from build123d import *

# Parameters (mm, degrees)
SKETCH007_R             = 3.5
SKETCH007_W             = 40
SKETCH007_H             = 65
PAD003_DEPTH            = 2
SKETCH017_W             = 44
SKETCH017_H             = 76
SKETCH017_W_2           = 40
SKETCH017_H_2           = 65
PAD009_DEPTH            = 12
SKETCH018_R             = 1
POCKET003_DEPTH         = 44
CHAMFER003_SIZE         = 5
CHAMFER004_SIZE         = 4
FILLET012_R             = 5
FILLET013_R             = 7
FILLET014_R             = 2
BODY001_ROLL_ANGLE      = 90
BODY001_PLACEMENT_ANGLE = 180


with BuildPart() as part:
    # Sketch007 → Pad003 (new body)
    with BuildSketch(Plane.XZ):
        Polygon((-5, 30), (5, 30), (43.613469, 5), (43.613469, -58), (47, -58), (47, -82), (-47, -82), (-47, -58), (-43.613469, -58), (-43.613469, 5), align=None)
        with Locations((0, -76)):
            Circle(SKETCH007_R, mode=Mode.SUBTRACT)
        with Locations((0, -29.5)):
            Rectangle(SKETCH007_W, SKETCH007_H, mode=Mode.SUBTRACT)
    extrude(amount=PAD003_DEPTH)

    # Sketch017 (on Face16 of Pad003) → Pad009 (join)
    with BuildSketch(Plane(origin=(0, 0, 0), x_dir=(1, 0, 0), z_dir=(0, 1, 0))):
        with Locations((0, 26)):
            Rectangle(SKETCH017_W, SKETCH017_H)
        with Locations((0, 29.5)):
            Rectangle(SKETCH017_W_2, SKETCH017_H_2, mode=Mode.SUBTRACT)
    extrude(amount=PAD009_DEPTH)

    # Sketch018 (on Face13 of Pad009) → Pocket003 (cut)
    with BuildSketch(Plane(origin=(-22, 0, 0), x_dir=(0, 0, -1), z_dir=(-1, 0, 0))):
        with Locations((32, -6.5)):
            Circle(SKETCH018_R)
    extrude(amount=-POCKET003_DEPTH, mode=Mode.SUBTRACT)

    # Chamfer003
    chamfer003_edges = [part.edges().sort_by_distance(p)[0] for p in [
        (0, 12, 12),
    ]]
    chamfer(chamfer003_edges, length=CHAMFER003_SIZE)

    # Chamfer004
    chamfer004_edges = [part.edges().sort_by_distance(p)[0] for p in [
        (0, 7, 12),
    ]]
    chamfer(chamfer004_edges, length=CHAMFER004_SIZE)

    # Fillet012
    fillet012_edges = [part.edges().sort_by_distance(p)[0] for p in [
        (0, 3, 12),
        (0, 9.828427, 9.171573),
        (0, 12, 7),
        (-22, 10.914214, 8.085786),
        (-22, 6.414214, 10.585786),
        (-22, 1.5, 12),
        (22, 10.914214, 8.085786),
        (22, 6.414214, 10.585786),
        (22, 1.5, 12),
    ]]
    fillet(fillet012_edges, radius=FILLET012_R)

    # Fillet013
    fillet013_edges = [part.edges().sort_by_distance(p)[0] for p in [
        (47, -1, -82),
        (-47, -1, -82),
    ]]
    fillet(fillet013_edges, radius=FILLET013_R)

    # Fillet014
    fillet014_edges = [part.edges().sort_by_distance(p)[0] for p in [
        (0, 0, -64),
        (0, 0, 12),
    ]]
    fillet(fillet014_edges, radius=FILLET014_R)


with BuildPart() as part_1:
    # Body001 roll: moved
    add(part.part.rotate(Axis((0, 0, 0), (1, 0, 0)), BODY001_ROLL_ANGLE))


with BuildPart() as part_2:
    # Body001 placement: moved
    add(part_1.part.moved(Location((0, 0, 31))).rotate(Axis((0, 0, 31), (0, 0, 1)), BODY001_PLACEMENT_ANGLE))


solid = part_2.part
Verification items for the finished model (mm, model axes). A direction names the side the tool comes from. Round coordinates to 2 decimals unless told otherwise and drop trailing zeros. Loops run counter-clockwise (first coordinate to the right, second up) from the corner with the lowest first, then second, coordinate; pieces in that order, holes last. Notation, with made-up numbers: (-3, 38.25) - (48, 38.25) arc R25 cw to (48, 76.25) - close; hole circle Ø2 at (72, 84). An arc over 180 degrees is marked (long way). Use one line per item in the form item = value.
1. Scan lines: probe 1 along Y at (x, z) = (0, 30.35); probe 2 along X at (y, z) = (-15.5, 33.75); probe 3 along Z at (x, y) = (-21, -32). Record each from-to range of solid material in increasing order.
A:
probe_1 = -82 to -79.5, -72.5 to -62, 3 to 30
probe_2 = -22 to -20, 20 to 22
probe_3 = 29 to 36.5, 38.5 to 43
2. Access from +Z, -Z, +X, -X, +Y, -Y to the whole of each face (thin tool, end or side, straight path). Record for faces 1 (the flat face through (22, -28, 38)), 2 (the flat face through (-22, -28, 38)), 3 (the cylindrical face through (20.574, 9.182, 36.874)), 4 (the flat face through (0, -62, 36)), 5 (the flat face through (0, -64, 38)).
A:
face_1 = +Z, +X, +Y, -Y
face_2 = +Z, -X, +Y, -Y
face_3 = +Z, +X, +Y
face_4 = +Z, -Z
face_5 = +Z, +X, -X, -Y
3. Draft check along Y on faces 6 (the cylindrical face through (21.127, 5.504, 41.417)), 7 (the cylindrical face through (0.759, -79.417, 30.014)), 8 (the flat face through (21, -30, 43)), 9 (the flat face through (20, -29, 36)). Enter one of: pulls with the +Y half, pulls with the -Y half, needs draft (parallel to the pull), parting line crosses it, or undercut.
A:
face_6 = pulls with the +Y half
face_7 = undercut
face_8 = needs draft
face_9 = undercut
4. Gauge pin test, flat ends, axial feed: pin 1 Ø4 at (x, z) = (23.5, 34) entering from -Y; pin 2 Ø3 at (y, z) = (-30, 38) entering from -X; pin 3 Ø8 at (y, z) = (7, 31) entering from -X. Record the tip position at first contact, or that the pin passes through.
A:
pin_1 = -64.03
pin_2 = -22
pin_3 = -43.61
5. Section check A-A on y = -14. Record the cut outline in (x, z).
A:
outline = (-43.61, 29) - (-20, 29) - (-20, 43) - (-22, 43) - (-22, 33) arc R2 cw to (-24, 31) - (-43.61, 31) - close; (20, 29) - (43.61, 29) - (43.61, 31) - (24, 31) arc R2 cw to (22, 33) - (22, 43) - (20, 43) - close
6. Section check D-D on x = -26.5. Record the cut outline in (y, z).
A:
outline = (-82, 29) - (16.08, 29) - (16.08, 31) - (-82, 31) - close
7. Section check B-B on x = 0. Give the number of separate pieces and of enclosed holes in the cut face, and give its area (3 significant figures).
A:
separate_pieces = 3
enclosed_holes = 0
area = 195 mm²
